For this review, take the finished solid that the model builds, in its own axes (mm). A direction names the side the tool comes from. Coordinates: 2 decimals unless noted, no trailing zeros. Write each loop counter-clockwise with the first axis right and the second up, starting at its lowest first coordinate (ties: lowest second). Pieces come first, ordered by that corner, then holes. Notation, with made-up numbers: (52, 76.5) -> (103, 76.5) arc R6 ccw to (103, 84.5) -> close; hole circle Ø8 at (-31, 54.5). An arc over 180 degrees is marked (long way). One line per item, written item: value. Start each with the question number.
1) Mouldability with a two-part tool opening along X and no side actions: class faces 3 (the flat face through (-20, 38.1, -1)), 4 (the flat face through (-39.688, 19, 3)), 5 (the flat face through (44.45, 16, 1)) as released by +X, released by -X, zero draft, split by the parting line, or undercut.
2) For pin 1 Ø1.5 at (x, y) = (3, 28.5) entering from +Z; pin 2 Ø8.5 at (x, z) = (34, -2) entering from +Y, all flat-tipped, find the tip position at first contact; note any pin that passes through.
3) For probe 1 along Y at (x, z) = (33, 47.5); probe 2 along Z at (x, y) = (-10, 6), list the stretches that pass through material, from the lowest coordinate up. Write a range as from..to.
4) Add section C-C (x = 8). State the section outline as (y, z) points.
5) Machinability: for faces 1 (the flat face through (1, -6.35, 1)), 2 (the flat face through (-10, 0, 3)), which of the approach directions +Z, -Z, +X, -X, +Y, -Y give a long, thin tool a straight path to every point of the face, cutting with its end or side? Answer none if there is none.
Autodesk Inventor part; units mm, degrees
ref_plane "YZ Plane" through (0, 0, 0) normal (1, 0, 0) x (0, 1, 0)
ref_plane "XZ Plane" through (0, 0, 0) normal (0, 1, 0) x (-1, 0, 0)
ref_plane "XY Plane" through (0, 0, 0) normal (0, 0, 1) x (1, 0, 0)
sketch "Sketch2" plane through (0, 0, 0) normal (0, 1, 0) x (-1, 0, 0)
  line L0 (44.45, 63.5) -> (-44.45, 63.5)
  line L1 (-44.45, 63.5) -> (-44.45, -63.5)
  line L2 (-44.45, -63.5) -> (44.45, -63.5)
  line L3 (44.45, -63.5) -> (44.45, 63.5)
  line L4 (44.45, 63.5) -> (-44.45, -63.5) construction
  line L5 (-44.45, 63.5) -> (44.45, -63.5) construction
  point P0 (0, 0)
  dimension "d0" = 127
  dimension "d1" = 88.9
extrude "Extrusion1" add sketch "Sketch2" against normal blind 6.35
sketch "Sketch4" plane through (0, 0, 0) normal (0, 1, 0) x (1, 0, 0)
  line L0 (-44.45, -63.5) -> (-44.45, 63.5)
  line L1 (44.45, 63.5) -> (44.45, -63.5)
  line L2 (-44.45, 63.5) -> (44.45, 63.5)
  line L3 (44.45, 63.5) -> (44.45, 58.7375)
  line L4 (44.45, 58.7375) -> (-44.45, 58.7375)
  line L5 (-44.45, 58.7375) -> (-44.45, 63.5)
  point P0 (0, 0)
  point P1 (-44.45, 58.7375)
  dimension "d4" = 4.7625
extrude "Extrusion2" add sketch "Sketch4" along normal blind 38.1
sketch "Sketch5" plane through (0, 0, 0) normal (0, 1, 0) x (1, 0, 0)
  line L0 (44.45, -63.5) -> (-44.45, -63.5)
  line L1 (-44.45, 58.7375) -> (44.45, 58.7375)
  line L2 (-44.45, -63.5) -> (-39.6875, -63.5)
  line L3 (-39.6875, -63.5) -> (-39.6875, 58.7375)
  line L4 (-44.45, 58.7375) -> (-44.45, -63.5)
  line L5 (44.45, 63.5) -> (44.45, -63.5)
  line L6 (44.45, -63.5) -> (39.6875, -63.5)
  line L7 (39.6875, -63.5) -> (39.6875, 58.7375)
  line L8 (44.45, 58.7375) -> (44.45, -63.5)
  line L9 (-44.45, 58.7375) -> (-44.45, -63.5)
  line L10 (-44.45, -63.5) -> (-44.45, 63.5)
  line L11 (-44.45, 58.7375) -> (-44.45, 63.5)
  line L12 (-44.45, 63.5) -> (-39.6875, 63.5)
  line L13 (-44.45, 63.5) -> (44.45, 63.5)
  line L14 (-39.6875, 58.7375) -> (-39.6875, 63.5)
  line L15 (44.45, 58.7375) -> (-44.45, 58.7375)
  line L16 (44.45, 58.7375) -> (44.45, 63.5)
  line L17 (39.6875, 63.5) -> (39.6875, 58.7375)
  point P0 (0, 0)
  point P1 (39.6875, -63.5)
  point P2 (-44.45, 58.7375)
  dimension "d7" = 4.7625
  dimension "d8" = 4.7625
extrude "Extrusion3" add sketch "Sketch5" along normal blind 38.1 contours L0 L7 L1 L5 | L1 L17 L13 L5 | L0 L4 L1 L3 | L1 L10 L12 L14
sketch "Sketch6" plane through (0, 0, 0) normal (0, 1, 0) x (1, 0, 0)
  line L0 (-39.6875, -63.5) -> (39.6875, -63.5)
  line L1 (-39.6875, 58.7375) -> (39.6875, 58.7375)
  line L2 (-22.225, -63.5) -> (-19.05, -63.5)
  line L3 (-19.05, -63.5) -> (-19.05, 58.7375)
  line L4 (-19.05, 58.7375) -> (-22.225, 58.7375)
  line L5 (-22.225, 58.7375) -> (-22.225, -63.5)
  line L6 (-1.5875, -63.5) -> (1.5875, -63.5)
  line L7 (1.5875, -63.5) -> (1.5875, 58.7375)
  line L8 (1.5875, 58.7375) -> (-1.5875, 58.7375)
  line L9 (-1.5875, 58.7375) -> (-1.5875, -63.5)
  line L10 (19.05, -63.5) -> (22.225, -63.5)
  line L11 (22.225, -63.5) -> (22.225, 58.7375)
  line L12 (22.225, 58.7375) -> (19.05, 58.7375)
  line L13 (19.05, 58.7375) -> (19.05, -63.5)
  line L14 (-39.6875, -63.5) -> (-39.6875, 58.7375)
  line L15 (39.6875, 58.7375) -> (39.6875, -63.5)
  point P0 (0, 0)
  point P1 (19.05, -63.5)
  point P2 (22.225, -63.5)
  point P3 (22.225, 58.7375)
  point P4 (-1.5875, 58.7375)
  point P5 (-1.5875, -63.5)
  dimension "d11" = 3.175
  dimension "d12" = 3.175
  dimension "d13" = 3.175
  dimension "d14" = 17.4625
  dimension "d15" = 17.4625
  dimension "d16" = 17.4625
  dimension "d17" = 17.4625
extrude "Extrusion4" add sketch "Sketch6" along normal blind 38.1 contours L5 L1 L3 L0 | L9 L1 L7 L0 | L13 L1 L11 L0
sketch "Sketch7" plane through (-39.6875, 0, -58.7375) normal (0, 0, 1) x (1, 0, 0)
  line L0 (0, 76.2) -> (0, 0) construction
  line L1 (0, 38.1) -> (79.375, 38.1) construction
  line L2 (79.375, 0) -> (79.375, 76.2) construction
  line L3 (39.6875, 38.1) -> (39.6875, 38.1) construction
  line L4 (84.1375, 38.1) -> (-4.7625, 38.1) construction
  point P0 (39.6875, 0)
  point P1 (8.7313, 38.1)
  point P2 (84.1375, 25.4)
  point P3 (-4.7625, 25.4)
  point P4 (8.7312, 38.1)
  dimension "d18" = 8.7312
equation "\"d0\" = depth"
equation "\"d1\" = width"
equation "\"d2\" = baseThickness"
equation "\"d4\" = backThickness"
equation "\"d5\" = backHeight"
equation "\"d7\" = edgeThickness"
equation "\"d8\" = edgeThickness"
equation "\"d9\" = edgeHeight"
equation "\"d11\" = dividerThickness"
equation "\"d12\" = dividerThickness"
equation "\"d13\" = dividerThickness"
equation "\"d14\" = dividerGap"
equation "\"d15\" = dividerGap"
equation "\"d16\" = dividerGap"
equation "\"d19\" = dividerHeight"
equation "\"baseThickness\" = 6.35"
equation "\"width\" = 88.9"
equation "\"depth\" = 127"
equation "\"backHeight\" = 38.1"
equation "\"backThickness\" = 4.7625"
equation "\"edgeThickness\" = 4.7625"
equation "\"edgeHeight\" = 38.1"
equation "\"dividerThickness\" = 3.175"
equation "\"dividerHeight\" = 38.1"
properties part number "shelfForElectronics"
Numbers:
1. face 3: zero draft
1. face 4: undercut
1. face 5: released by +X
2. pin 1: z = -58.74
2. pin 2: y = 0
3. probe 1: -6.35..0
3. probe 2: -63.5..-58.74
4. outline: (-6.35, -63.5) -> (38.1, -63.5) -> (38.1, -58.74) -> (0, -58.74) -> (0, 63.5) -> (-6.35, 63.5) -> close
5. face 1: +Z, -Z, +X, -X, -Y
5. face 2: +Z, +Y
